from build123d import *

# Parameters (mm, degrees)
SKETCH1_W           = 145
SKETCH1_H           = 90
BOSS_EXTRUDE1_DEPTH = 1.5
SKETCH2_W           = 149
SKETCH2_H           = 94
SKETCH2_W_2         = 145
SKETCH2_H_2         = 90
BOSS_EXTRUDE2_DEPTH = 8
SKETCH3_W           = 147
SKETCH3_H           = 92
SKETCH3_W_2         = 145
SKETCH3_H_2         = 90
CUT_EXTRUDE1_DEPTH  = 1.5


with BuildPart() as part:
    # Sketch1 → Boss-Extrude1 (new body)
    with BuildSketch(Plane(origin=(0, 0, 0), x_dir=(1, 0, 0), z_dir=(0, 1, 0))):
        Rectangle(SKETCH1_W, SKETCH1_H)
    extrude(amount=BOSS_EXTRUDE1_DEPTH)

    # Sketch2 → Boss-Extrude2 (add)
    with BuildSketch(Plane(origin=(0, 0, 0), x_dir=(1, 0, 0), z_dir=(0, 1, 0))):
        Rectangle(SKETCH2_W, SKETCH2_H)
        Rectangle(SKETCH2_W_2, SKETCH2_H_2, mode=Mode.SUBTRACT)
    extrude(amount=BOSS_EXTRUDE2_DEPTH)

    # Sketch3 → Cut-Extrude1 (cut)
    with BuildSketch(Plane(origin=(0, 8, 0), x_dir=(1, 0, 0), z_dir=(0, 1, 0))):
        Rectangle(SKETCH3_W, SKETCH3_H)
        Rectangle(SKETCH3_W_2, SKETCH3_H_2, mode=Mode.SUBTRACT)
    extrude(amount=-CUT_EXTRUDE1_DEPTH, mode=Mode.SUBTRACT)


solid = part.part
Work out the finished part from the listing and answer in its coordinate system (mm). A direction names the side the tool comes from. Give positions to 0.01 mm unless a question says otherwise; leave off trailing zeros. Loops run counter-clockwise (first coordinate to the right, second up) from the corner with the lowest first, then second, coordinate; pieces in that order, holes last. Notation, with made-up numbers: (-35, 21.5) -> (-25, 21.5) arc R15 cw to (-25, 40.5) -> close; hole circle Ø3 at (-34, -11.5). An arc over 180 degrees is marked (long way). Use a Markdown table: item, result. Add a question column.
1. A flat-ended cylindrical pin translates along its axis: pin 1 Ø10 at (x, z) = (-38.5, -18.5) entering from +Y. Find the tip coordinate at first contact, or state that the pin passes through.
2. Section B-B on x = 14 is taken. Determine the outline of the cut face in (y, z).
3. Determine the mould class of faces 1 (the flat face through (74.5, 4, 1)), 2 (the flat face through (-1, 4, -47)), 3 (the flat face through (-1, 4, 45)) for opening direction Z: released by +Z, released by -Z, zero draft, split by the parting line, or undercut.
4. Section A-A on y = 3.5 is taken. Determine the outline of the cut face in (x, z), and give its area (3 significant figures).
5. For faces 4 (the flat face through (72.5, 4, 1)), 5 (the flat face through (-74.5, 4, 1)), determine the directions among +Z, -Z, +X, -X, +Y, -Y from which every point of the face is accessible in a straight line to the end or side of a thin tool.
6. Section C-C on z = 19 is taken. Determine the outline of the cut face in (x, y).
7. Find the intervals of material crossed by probe 1 along Z at (x, y) = (-53, 5); probe 2 along X at (y, z) = (4, 26.5); probe 3 along Z at (x, y) = (5, 7), in increasing order.
Results below:
| question | item | result |
|---|---|---|
| 1 | pin 1 | stops at y = 1.5 |
| 2 | outline | (0, -47) -> (8, -47) -> (8, -46) -> (6.5, -46) -> (6.5, -45) -> (1.5, -45) -> (1.5, 45) -> (6.5, 45) -> (6.5, 46) -> (8, 46) -> (8, 47) -> (0, 47) -> close |
| 3 | face 1 | zero draft |
| 3 | face 2 | released by -Z |
| 3 | face 3 | undercut |
| 4 | outline | (-74.5, -47) -> (74.5, -47) -> (74.5, 47) -> (-74.5, 47) -> close; hole (-72.5, -45) -> (72.5, -45) -> (72.5, 45) -> (-72.5, 45) -> close |
| 4 | area | 956 mm^2 |
| 5 | face 4 | +Y |
| 5 | face 5 | +Z, -Z, -X, +Y, -Y |
| 6 | outline | (-74.5, 0) -> (74.5, 0) -> (74.5, 8) -> (73.5, 8) -> (73.5, 6.5) -> (72.5, 6.5) -> (72.5, 1.5) -> (-72.5, 1.5) -> (-72.5, 6.5) -> (-73.5, 6.5) -> (-73.5, 8) -> (-74.5, 8) -> close |
| 7 | probe 1 | z = -47 to -45, 45 to 47 |
| 7 | probe 2 | x = -74.5 to -72.5, 72.5 to 74.5 |
| 7 | probe 3 | z = -47 to -46, 46 to 47 |
